Could you check a few things on this model? Use its own coordinates, in mm. Round coordinates to 2 decimals unless told otherwise and drop trailing zeros. Write each loop counter-clockwise with the first axis right and the second up, starting at its lowest first coordinate (ties: lowest second). Pieces come first, ordered by that corner, then holes. Notation, with made-up numbers: M -12.75,-10.5 L 25.25,-10.5 A20 ccw 25.25,-1.5 Z; hole C 80.5,14 d1. An arc over 180 degrees is marked long. One line per item, written item: value. Start each with the question number.
(1) I want a section at C-C on z = 0. Please give me the cut outline in (x, y).
(2) If I drill on L1, parallel to X at y = -0.6, z = 0; L2, parallel to X at y = -1.35, z = 1.75; L3, parallel to Z at x = -68, y = -1.6, over which ranges is the centre line in solid material (lowest first)?
(3) I want a section at A-A on x = -50. Please give me the cut outline in (y, z).
(4) Thinking about a two-plate mould opening in X: for faces 1 (the face through (10, -1, 0)), 2 (the face through (-34, -2.5, 0)), 3 (the face through (-47.95, -0.49, -0.65)), which applies, released by +X, released by -X, zero draft, split by the parting line, or undercut?
(5) I want a section at B-B on y = -0.55. Please give me the cut outline in (x, z), and give its area (3 significant figures).
(6) I want a section at D-D on z = 8.75. Please give me the cut outline in (x, y).
(7) I'm going to push flat-ended pins straight in: pin 1 Ø2.5 at (x, z) = (-50, 0) entering from +Y; pin 2 Ø1 at (y, z) = (-0.5, -7) entering from -X; pin 3 Ø5 at (x, z) = (-20, 0) entering from -Y; pin 4 Ø1.5 at (y, z) = (-1.5, 6.5) entering from -X. Where does each tip first touch, or does it pass through?
```python
from build123d import *

# Parameters (mm, degrees)
SKETCH1_R             = 2.15
BOSS_EXTRUDE1_DEPTH   = 2.5
CHAMFER1_SIZE         = 1.5
CHAMFER1_SIZE2        = 2.598076211
CHAMFER1_PART_2_SIZE  = 1.5
CHAMFER1_PART_2_SIZE2 = 2.598076211
CHAMFER1_PART_3_SIZE  = 1.5
CHAMFER1_PART_3_SIZE2 = 2.598076211
CHAMFER1_PART_4_SIZE  = 1.5
CHAMFER1_PART_4_SIZE2 = 2.598076211


with BuildPart() as part:
    # Sketch1 → Boss-Extrude1 (new body)
    with BuildSketch(Plane(origin=(0, 0, 0), x_dir=(1, 0, 0), z_dir=(0, 1, 0))):
        with BuildLine():
            Line((0, -10), (-70, -10))
            ThreePointArc((-70, -10), (-80, 0), (-70, 10))
            Line((-70, 10), (0, 10))
            ThreePointArc((0, 10), (10, 0), (0, -10))
        make_face()
        Circle(SKETCH1_R, mode=Mode.SUBTRACT)
        with Locations((-70, 0)):
            Circle(SKETCH1_R, mode=Mode.SUBTRACT)
        with Locations((-20, 0)):
            Circle(SKETCH1_R, mode=Mode.SUBTRACT)
        with Locations((-50, 0)):
            Circle(SKETCH1_R, mode=Mode.SUBTRACT)
    extrude(amount=-BOSS_EXTRUDE1_DEPTH)

    # Chamfer1
    chamfer1_edges = [part.edges().sort_by_distance(p)[0] for p in [
        (-2.15, -2.5, 0),
    ]]
    chamfer1_side = [part.faces().sort_by_distance(p)[0] for p in [
        (-2.15, -1.25, 0),
    ]]
    chamfer(chamfer1_edges, length=CHAMFER1_SIZE, length2=CHAMFER1_SIZE2, reference=chamfer1_side[0])

    # Chamfer1 part 2
    chamfer1_part_2_edges = [part.edges().sort_by_distance(p)[0] for p in [
        (-72.15, -2.5, 0),
    ]]
    chamfer1_part_2_side = [part.faces().sort_by_distance(p)[0] for p in [
        (-72.15, -1.25, 0),
    ]]
    chamfer(chamfer1_part_2_edges, length=CHAMFER1_PART_2_SIZE, length2=CHAMFER1_PART_2_SIZE2, reference=chamfer1_part_2_side[0])

    # Chamfer1 part 3
    chamfer1_part_3_edges = [part.edges().sort_by_distance(p)[0] for p in [
        (-22.15, -2.5, 0),
    ]]
    chamfer1_part_3_side = [part.faces().sort_by_distance(p)[0] for p in [
        (-22.15, -1.25, 0),
    ]]
    chamfer(chamfer1_part_3_edges, length=CHAMFER1_PART_3_SIZE, length2=CHAMFER1_PART_3_SIZE2, reference=chamfer1_part_3_side[0])

    # Chamfer1 part 4
    chamfer1_part_4_edges = [part.edges().sort_by_distance(p)[0] for p in [
        (-52.15, -2.5, 0),
    ]]
    chamfer1_part_4_side = [part.faces().sort_by_distance(p)[0] for p in [
        (-52.15, -1.25, 0),
    ]]
    chamfer(chamfer1_part_4_edges, length=CHAMFER1_PART_4_SIZE, length2=CHAMFER1_PART_4_SIZE2, reference=chamfer1_part_4_side[0])


solid = part.part
```
Found:
1. outline: M -80,-2.5 L -74.75,-2.5 L -72.15,-1 L -72.15,0 L -80,0 Z; M -67.85,-1 L -65.25,-2.5 L -54.75,-2.5 L -52.15,-1 L -52.15,0 L -67.85,0 Z; M -47.85,-1 L -45.25,-2.5 L -24.75,-2.5 L -22.15,-1 L -22.15,0 L -47.85,0 Z; M -17.85,-1 L -15.25,-2.5 L -4.75,-2.5 L -2.15,-1 L -2.15,0 L -17.85,0 Z; M 2.15,-1 L 4.75,-2.5 L 10,-2.5 L 10,0 L 2.15,0 Z
2. L1: x = -80 to -72.15, -67.85 to -52.15, -47.85 to -22.15, -17.85 to -2.15, 2.15 to 10
2. L2: x = -79.85 to -72.13, -67.87 to -52.13, -47.87 to -22.13, -17.87 to -2.13, 2.13 to 9.85
2. L3: z = -10 to -2.48, 2.48 to 10
3. outline: M -2.5,-10 L 0,-10 L 0,-2.15 L -1,-2.15 L -2.5,-4.75 Z; M -2.5,4.75 L -1,2.15 L 0,2.15 L 0,10 L -2.5,10 Z
4. face 1: released by +X
4. face 2: zero draft
4. face 3: undercut
5. outline: M -70,-10 L 0,-10 A10 ccw 0,10 L -70,10 A10 ccw Z; hole C -70,0 d4.3; hole C -50,0 d4.3; hole C -20,0 d4.3; hole C 0,0 d4.3
5. area: 1,660 mm²
6. outline: M -74.84,-2.5 L 4.84,-2.5 L 4.84,0 L -74.84,0 Z
7. pin 1: passes through
7. pin 2: stops at x = -77.6
7. pin 3: stops at y = -1.2
7. pin 4: stops at x = -78.18
